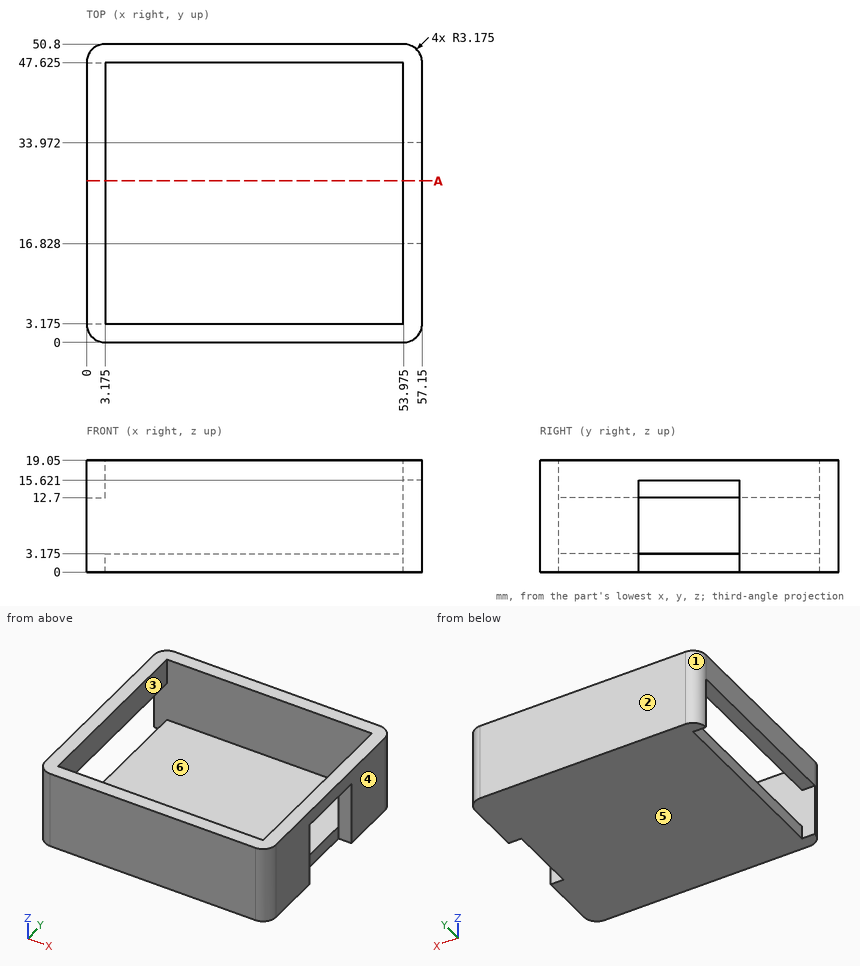
The drawing under review shows one solid part. Ordinate dimensions are in mm from its lowest x, y, z. A direction names the side the tool comes from. Round coordinates to 2 decimals unless told otherwise and drop trailing zeros. Use a Markdown table: item, result. Add a question column.
Q1. Machinability: for the marked faces 5 and 6, which of the approach directions +Z, -Z, +X, -X, +Y, -Y give a long, thin tool a straight path to every point of the face, cutting with its end or side? Answer none if there is none.
Q2. Add section A-A (y = 27.5). State how many separate pieces and enclosed holes the cut face has, plus the area to 3 significant figures.
Q3. The part is to be moulded in two halves that separate along X. For the marked faces 1, 2, 3 and 4, say which applies: pulls with the +X half, pulls with the -X half, needs draft (parallel to the pull), parting line crosses it, or undercut.
Q4. For probe 1 along Y at (x, z) = (19.5, 11) (1 decimal); probe 2 along Z at (x, y) = (30, 11.5) (1 decimal), list the stretches that pass through material, from the lowest coordinate up.
Q5. Insertion check: pin 1 Ø13.5 at (x, y) = (40.5, 18.5) entering from +Z (1 decimal); pin 2 Ø1 at (x, z) = (55, 6.5) entering from -Y; pin 3 Ø1.6 at (x, y) = (2, 30) entering from -Z. Each pin has a flat end and moves straight along its axis. Give the tip position at first contact, or say it passes through.
Worked answers:
| question | item | result |
|---|---|---|
| 1 | face 5 | -Z, +X, -X, +Y, -Y |
| 1 | face 6 | +Z, -X |
| 2 | separate pieces | 3 |
| 2 | enclosed holes | 0 |
| 2 | area | 192 mm² |
| 3 | face 1 | pulls with the -X half |
| 3 | face 2 | needs draft |
| 3 | face 3 | undercut |
| 3 | face 4 | pulls with the +X half |
| 4 | probe 1 | 0 to 3.2, 47.6 to 50.8 |
| 4 | probe 2 | 0 to 3.2 |
| 5 | pin 1 | z = 3.2 |
| 5 | pin 2 | y = 0.04 |
| 5 | pin 3 | z = 12.7 |
